Build history of the part. All positions in model axes, mm. Face numbers are marked on the shaded views. A direction names the side the tool comes from. Round coordinates to 2 decimals unless told otherwise and drop trailing zeros. Write each loop counter-clockwise with the first axis right and the second up, starting at its lowest first coordinate (ties: lowest second). Pieces come first, ordered by that corner, then holes. Notation, with made-up numbers: (50, -13.75) -> (57, -13.75) arc R28 ccw to (57, 9.25) -> close; hole circle Ø11 at (47.25, 31). An arc over 180 degrees is marked (long way). Return JSON: item names as keys, results as strings.
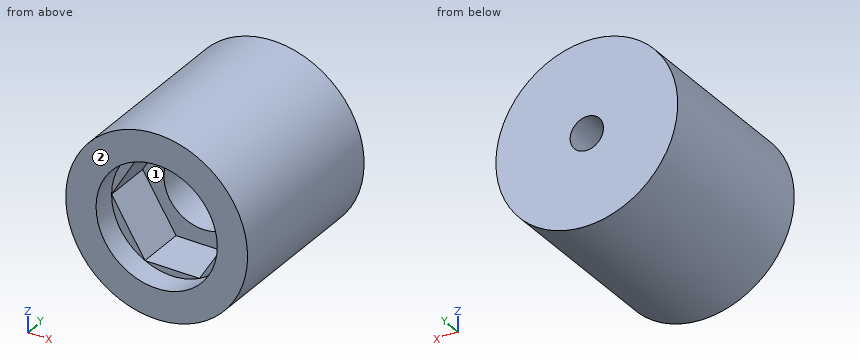
from build123d import *

# Parameters (mm, degrees)
F0_R     = 15
F0_R_2   = 9.25
F0_R_3   = 4.5
F0_R_4   = 2.75
F1_DEPTH = 30
F2_R     = 10
F2_R_2   = 2.75
F3_DEPTH = 12
F4_R     = 6.5
F4_R_2   = 2.75
F5_DEPTH = 12
F7_DEPTH = 8


with BuildPart() as f1:
    # F0 (on Front) → F1 (new body)
    with BuildSketch(Plane.XZ):
        Circle(F0_R)
        Circle(F0_R_2, mode=Mode.SUBTRACT)
        Circle(F0_R_2)
        Circle(F0_R_3, mode=Mode.SUBTRACT)
        Circle(F0_R_3)
        Circle(F0_R_4, mode=Mode.SUBTRACT)
    extrude(amount=F1_DEPTH)

    # F2 (on face) → F3 (cut)
    with BuildSketch(Plane.XZ.offset(30)):
        Circle(F2_R)
        Circle(F2_R_2, mode=Mode.SUBTRACT)
    extrude(amount=-F3_DEPTH, mode=Mode.SUBTRACT)

    # F4 (on face) → F5 (cut)
    with BuildSketch(Plane.XZ.offset(18)):
        Circle(F4_R)
        Circle(F4_R_2, mode=Mode.SUBTRACT)
    extrude(amount=-F5_DEPTH, mode=Mode.SUBTRACT)

    # F6 (on face) → F7 (join)
    with BuildSketch(Plane.XZ.offset(18)):
        with BuildLine():
            ThreePointArc((4.4908489249, 8.9348909301), (-0.195068874, 9.9980972257), (-4.8359487164, 8.7529195137))
            Line((-4.8359487164, 8.7529195137), (4.4908489249, 8.9348909301))
        make_face()
        with BuildLine():
            ThreePointArc((10, 0), (8.5120059107, 5.2484050316), (4.4908489249, 8.9348909301))
            Line((4.4908489249, 8.9348909301), (10, 0))
        make_face()
        with BuildLine():
            ThreePointArc((4.4908489249, -8.9348909301), (8.5120059107, -5.2484050316), (10, 0))
            Line((10, 0), (4.4908489249, -8.9348909301))
        make_face()
        with BuildLine():
            Line((4.4908489249, -8.9348909301), (-4.4908489249, -8.9348909301))
            ThreePointArc((-4.4908489249, -8.9348909301), (0, -10), (4.4908489249, -8.9348909301))
        make_face()
        with BuildLine():
            Line((-4.4908489249, -8.9348909301), (-10, 0))
            ThreePointArc((-10, 0), (-8.5120059107, -5.2484050316), (-4.4908489249, -8.9348909301))
        make_face()
        with BuildLine():
            Line((-10, 0), (-4.8359487164, 8.7529195137))
            ThreePointArc((-4.8359487164, 8.7529195137), (-8.6127663141, 5.0813636377), (-10, 0))
        make_face()
    extrude(amount=F7_DEPTH)


solid = f1.part
Q1. 3-axis set-ups, long thin cutter, end or side, ignore diameter. For the marked faces 1 and 2: which of +Z, -Z, +X, -X, +Y, -Y reach the whole face in a straight line?
Verdict:
{"face 1": "-Y", "face 2": "+Z, -Z, +X, -X, -Y"}
Q2. Saw through at B-B on x = 0. List the corners of the cut face in (y, z), then the cut area to 3 significant figures.
Verdict:
{"outline": "(-30, -15) -> (0, -15) -> (0, -2.75) -> (-6, -2.75) -> (-6, -6.5) -> (-18, -6.5) -> (-18, -8.93) -> (-26, -8.93) -> (-26, -10) -> (-30, -10) -> close; (-30, 10) -> (-26, 10) -> (-26, 8.85) -> (-18, 8.85) -> (-18, 6.5) -> (-6, 6.5) -> (-6, 2.75) -> (0, 2.75) -> (0, 15) -> (-30, 15) -> close", "area": "489 mm²"}
Q3. Wall check: L1, parallel to Z at x = 0, y = -12.5; L2, parallel to Z at x = 0, y = -1.4; L3, parallel to Y at x = -4.75, z = 0.75. Give the ranges that are in metal, low to high.
Verdict:
{"L1": "z = -15 to -6.5, 6.5 to 15", "L2": "z = -15 to -2.75, 2.75 to 15", "L3": "y = -6 to 0"}
Q4. Saw through at A-A on y = -23.5. List the corners of the cut face in (x, z), then the cut area to 3 significant figures.
Verdict:
{"outline": "circle Ø30 at (0, 0); hole (-10, 0) -> (-4.49, -8.93) -> (4.49, -8.93) -> (10, 0) -> (4.49, 8.93) -> (-4.84, 8.75) -> close", "area": "448 mm²"}
Q5. Saw through at D-D on x = 5.75. List the corners of the cut face in (y, z).
Verdict:
{"outline": "(-30, -13.85) -> (0, -13.85) -> (0, 13.85) -> (-30, 13.85) -> (-30, 8.18) -> (-26, 8.18) -> (-26, 6.89) -> (-18, 6.89) -> (-18, 3.03) -> (-6, 3.03) -> (-6, -3.03) -> (-18, -3.03) -> (-18, -6.89) -> (-26, -6.89) -> (-26, -8.18) -> (-30, -8.18) -> close"}
Q6. Pin check, flat tips, straight feed: pin 1 Ø1.5 at (y, z) = (-25, -6) entering from +X; pin 2 Ø14.5 at (x, z) = (0, -1.5) entering from -Y; pin 3 Ø1 at (x, y) = (10.5, -4) entering from +Z. Stop position of each tip, or through.
Verdict:
{"pin 1": "stops at x = 14.05", "pin 2": "stops at y = -18", "pin 3": "stops at z = 11.18"}
Q7. Saw through at C-C on z = 7.25. List the corners of the cut face in (x, y).
Verdict:
{"outline": "(-13.13, -30) -> (-6.89, -30) -> (-6.89, -26) -> (-5.72, -26) -> (-5.72, -18) -> (5.53, -18) -> (5.53, -26) -> (6.89, -26) -> (6.89, -30) -> (13.13, -30) -> (13.13, 0) -> (-13.13, 0) -> close"}
